Job drawing, mm, ordinate dimensions from the low corner. One solid piece. Round coordinates to 2 decimals unless told otherwise and drop trailing zeros. Loops run counter-clockwise (first coordinate to the right, second up) from the corner with the lowest first, then second, coordinate; pieces in that order, holes last. Notation, with made-up numbers: M 5,8.5 L 49,8.5 A23 ccw 49,36.5 Z; hole C -32.75,75 d8. An arc over 180 degrees is marked long. One line per item, written item: value.
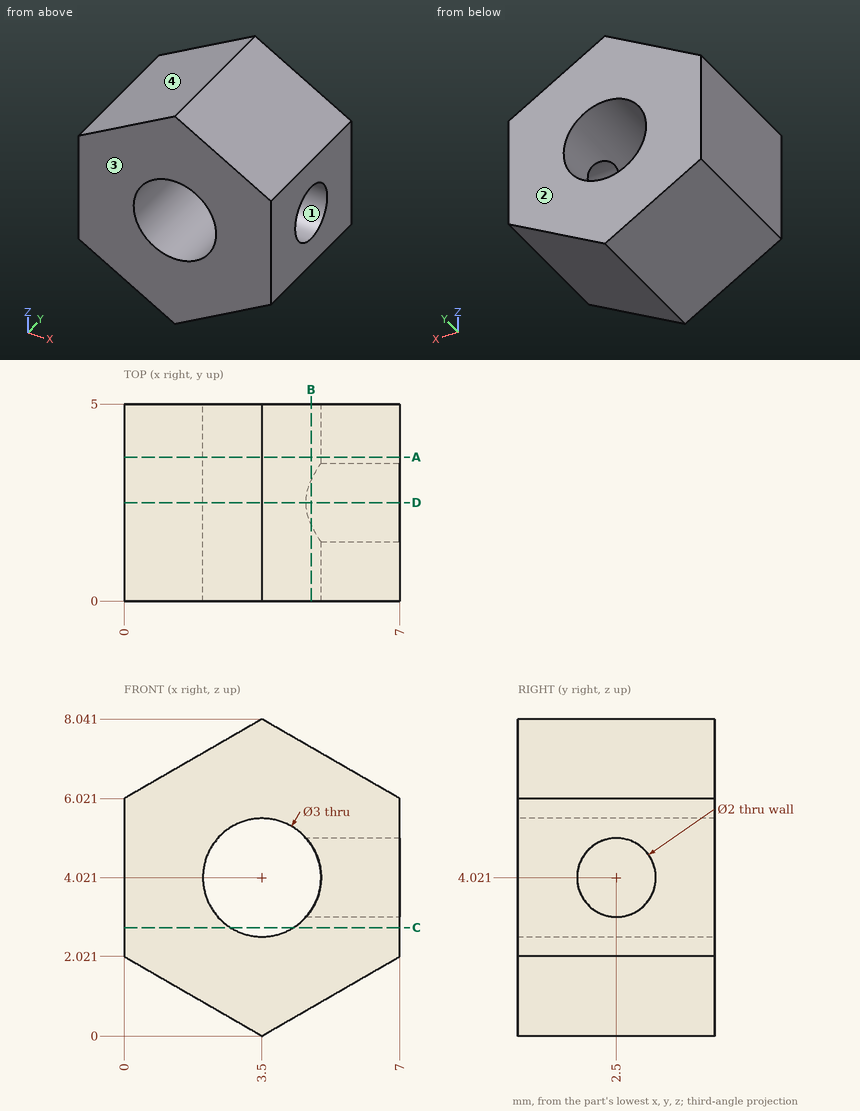
Item 1: Drop flat-ended pins along their axis: P1, Ø3, axis at x = 4.5, y = 3.5, coming from the +Z side; P2, Ø2.5, axis at x = 3.5, z = 4.02, coming from the +Y side; P3, Ø3, axis at x = 6, y = 3, coming from the +Z side (1 decimal). Give the stop position or say it passes through.
Check values:
P1: stops at z = 8.04
P2: passes through
P3: stops at z = 7.5
Item 2: Pull direction Y, two halves, no side cores. Call the marked faces 1, 2, 3 and 4: pulls with the +Y half, pulls with the -Y half, needs draft (parallel to the pull), parting line crosses it, or undercut.
Check values:
face 1: undercut
face 2: pulls with the +Y half
face 3: pulls with the -Y half
face 4: needs draft
Item 3: Wall check: line 1 along Z through (x, y) = (2.5, 2.75) (1 decimal); line 2 along X through (y, z) = (1.8, 4); line 3 along Z through (x, y) = (2.75, 3.7). Give the ranges that are in metal, low to high.
Check values:
line 1: z = 0.6 to 2.9, 5.1 to 7.5
line 2: x = 0 to 2
line 3: z = 0.43 to 2.72, 5.32 to 7.61
Item 4: Slice it at C-C, the plane z = 2.75. Give the cut face in (x, y).
Check values:
outline: M 0,0 L 2.7,0 L 2.7,5 L 0,5 Z; M 4.3,0 L 7,0 L 7,5 L 4.3,5 Z
Item 5: Slice it at A-A, the plane y = 3.65. Give the cut face in (x, z).
Check values:
outline: M 0,2.02 L 3.5,0 L 7,2.02 L 7,6.02 L 3.5,8.04 L 0,6.02 Z; hole C 3.5,4.02 d3
Item 6: Slice it at D-D, the plane y = 2.5. Give the cut face in (x, z).
Check values:
outline: M 0,2.02 L 3.5,0 L 7,2.02 L 7,3.02 L 4.62,3.02 A1.5 cw long 4.62,5.02 L 7,5.02 L 7,6.02 L 3.5,8.04 L 0,6.02 Z
Item 7: Slice it at B-B, the plane x = 4.75. Give the cut face in (y, z).
Check values:
outline: M 0,0.72 L 5,0.72 L 5,3.19 L 3.06,3.19 A1 cw 1.94,3.19 L 0,3.19 Z; M 0,4.85 L 1.94,4.85 A1 cw 3.06,4.85 L 5,4.85 L 5,7.32 L 0,7.32 Z
